Source: CAD feature listing. Evaluate the final solid. Frame: model axes, mm. A direction names the side the tool comes from. Coordinates: 2 decimals unless noted, no trailing zeros. Write each loop counter-clockwise with the first axis right and the second up, starting at its lowest first coordinate (ties: lowest second). Pieces come first, ordered by that corner, then holes. Notation, with made-up numbers: M 55.25,81.5 L 95.25,81.5 A23 cw 95.25,94.5 Z; hole C 34,79 d6. An arc over 180 degrees is marked long. One line per item, written item: value. Start each with the question number.
Item 1: Ray query, L1, parallel to Z at x = -23.5, y = 2; L2, parallel to X at y = 8.75, z = 14; L3, parallel to Y at x = 13, z = 19. Return the intervals inside material, ascending. Write a range as from..to.
Item 2: Cut plane A-A, the plane x = 19.5. Output: boundary loops of the cut face in (y, z), then the cut area to 3 significant figures.
Item 3: Cut plane C-C, the plane z = -12.5. Output: boundary loops of the cut face in (x, y).
Item 4: Pin query (flat end, axial travel): P1, Ø21, axis at x = 3.5, z = -9.5, coming from the -Y side. Return the tip coordinate at first contact, or that it passes through.
Item 5: Mould query, pull axis Z, two halves, no side actions, for faces 1 (the flat face through (0, 12, 25)), 2 (the cylindrical face through (-31.4, 26.43, 0.29)), 3 (the flat face through (-34, 12, 0)). Classes: released by +Z, released by -Z, zero draft, split by the parting line, or undercut.
Item 6: Set-up query: faces 4 (the flat face through (0, 27, 0)), 5 (the flat face through (34, 12, 0)). Return all of +Z, -Z, +X, -X, +Y, -Y with unobstructed straight access to the full face (end or side cutting, diameter ignored); none if empty.
Item 7: Cut plane B-B, the plane y = 24. Output: boundary loops of the cut face in (x, z), then the cut area to 3 significant figures.
Autodesk Inventor part; units mm, degrees
ref_plane "YZ Plane" through (0, 0, 0) normal (1, 0, 0) x (0, 1, 0)
ref_plane "XZ Plane" through (0, 0, 0) normal (0, 1, 0) x (-1, 0, 0)
ref_plane "XY Plane" through (0, 0, 0) normal (0, 0, 1) x (1, 0, 0)
sketch "Sketch1" plane through (0, 0, 0) normal (0, 1, 0) x (-1, 0, 0)
  line L0 (30, 25) -> (-30, 25)
  line L1 (-34, 21) -> (-34, -21)
  line L2 (-30, -25) -> (30, -25)
  line L3 (34, -21) -> (34, 21)
  line L4 (34, 25) -> (-34, -25) construction
  line L5 (-34, 25) -> (34, -25) construction
  arc A0 (30, -25) -> (34, -21) centre (30, -21) ccw
  arc A1 (34, 21) -> (30, 25) centre (30, 21) ccw
  arc A2 (-30, 25) -> (-34, 21) centre (-30, 21) ccw
  arc A3 (-34, -21) -> (-30, -25) centre (-30, -21) ccw
  point P0 (0, 0)
  dimension "d0" = 68
  dimension "d1" = 50
  dimension "d2" = 4
extrude "Extrusion1" add sketch "Sketch1" along normal blind 29
fillet "Fillet1" radius 4 8 edges at (32.8284, 29, 23.8284) (34, 29, 0) (32.8284, 29, -23.8284) (0, 29, -25) (-32.8284, 29, -23.8284) (-34, 29, 0) (-32.8284, 29, 23.8284) (0, 29, 25)
shell "Shell1" thickness 2 removed faces 1 at (10, 0, 8.3333)
properties part number "Fuse Box 6-way-lid" material "PMMA Plastic"
From the geometry:
1. L1: z = -25..-23, 23..25
1. L2: x = -34..-32, 32..34
1. L3: y = 27..29
2. outline: M 0,-25 L 25,-25 A4 ccw 29,-21 L 29,21 A4 ccw 25,25 L 0,25 L 0,23 L 25,23 A2 cw 27,21 L 27,-21 A2 cw 25,-23 L 0,-23 Z
2. area: 203 mm²
3. outline: M -34,0 L -32,0 L -32,25 A2 cw -30,27 L 30,27 A2 cw 32,25 L 32,0 L 34,0 L 34,25 A4 ccw 30,29 L -30,29 A4 ccw -34,25 Z
4. P1: stops at y = 27
5. face 1: released by +Z
5. face 2: undercut
5. face 3: zero draft
6. face 4: -Y
6. face 5: +Z, -Z, +X, +Y, -Y
7. outline: M -34,-21 A4 ccw -30,-25 L 30,-25 A4 ccw 34,-21 L 34,21 A4 ccw 30,25 L -30,25 A4 ccw -34,21 Z; hole M -32,-21 A2 ccw -30,-23 L 30,-23 A2 ccw 32,-21 L 32,21 A2 ccw 30,23 L -30,23 A2 ccw -32,21 Z
7. area: 446 mm²
